from build123d import *

# Parameters (mm, degrees)
F1_DEPTH = 1.2
F2_DEPTH = 4
F3_DEPTH = 3.5
F4_W     = 1.7
F4_H     = 3.5
F5_DEPTH = 0.2


# Not quite as in the source:
# - a feature names something its author has since deleted; it is built from what else it names


with BuildPart() as f1:
    # F0 (on Top) → F1 (new body)
    with BuildSketch(Plane.XY):
        with BuildLine():
            ThreePointArc((-10.7121426428, 2.5), (-10.5820537772, 3.0033544341), (-10.4283268073, 3.5))
            Line((-10.4283268073, 3.5), (-14.25, 3.5))
            Line((-14.25, 3.5), (-14.25, 2.5))
            Line((-14.25, 2.5), (-10.7121426428, 2.5))
        make_face()
        with BuildLine():
            ThreePointArc((-10.4283268073, -3.5), (-10.5820537772, -3.0033544341), (-10.7121426428, -2.5))
            Line((-10.7121426428, -2.5), (-14.25, -2.5))
            Line((-14.25, -2.5), (-14.25, -3.5))
            Line((-14.25, -3.5), (-10.4283268073, -3.5))
        make_face()
        with BuildLine():
            Line((-9.3722996111, -2.5), (-10.7121426428, -2.5))
            ThreePointArc((-10.7121426428, -2.5), (-10.5820537772, -3.0033544341), (-10.4283268073, -3.5))
            Line((-10.4283268073, -3.5), (-9.0465463023, -3.5))
            ThreePointArc((-9.0465463023, -3.5), (-9.2229860238, -3.004418214), (-9.3722996111, -2.5))
        make_face()
        with BuildLine():
            Line((-9.0465463023, 3.5), (-10.4283268073, 3.5))
            ThreePointArc((-10.4283268073, 3.5), (-10.5820537772, 3.0033544341), (-10.7121426428, 2.5))
            Line((-10.7121426428, 2.5), (-9.3722996111, 2.5))
            ThreePointArc((-9.3722996111, 2.5), (-9.2229860238, 3.004418214), (-9.0465463023, 3.5))
        make_face()
        with BuildLine():
            Line((-9.3722996111, 2.5), (-10.7121426428, 2.5))
            ThreePointArc((-10.7121426428, 2.5), (-11, 0), (-10.7121426428, -2.5))
            Line((-10.7121426428, -2.5), (-9.3722996111, -2.5))
            ThreePointArc((-9.3722996111, -2.5), (-9.7, 0), (-9.3722996111, 2.5))
        make_face()
        with BuildLine():
            ThreePointArc((9.0465463023, 3.5), (7.606386924, 6.0193752136), (5.4854352608, 8))
            Line((5.4854352608, 8), (5, 8))
            Line((5, 8), (3.5, 6.4))
            Line((3.5, 6.4), (-3.5, 6.4))
            Line((-3.5, 6.4), (-5, 8))
            Line((-5, 8), (-5.4854352608, 8))
            ThreePointArc((-5.4854352608, 8), (-7.606386924, 6.0193752136), (-9.0465463023, 3.5))
            Line((-9.0465463023, 3.5), (9.0465463023, 3.5))
        make_face()
        with BuildLine():
            ThreePointArc((9.3722996111, 2.5), (9.2229860238, 3.004418214), (9.0465463023, 3.5))
            Line((9.0465463023, 3.5), (-9.0465463023, 3.5))
            ThreePointArc((-9.0465463023, 3.5), (-9.2229860238, 3.004418214), (-9.3722996111, 2.5))
            ThreePointArc((-9.3722996111, 2.5), (-9.7, 0), (-9.3722996111, -2.5))
            ThreePointArc((-9.3722996111, -2.5), (-9.2229860238, -3.004418214), (-9.0465463023, -3.5))
            Line((-9.0465463023, -3.5), (9.0465463023, -3.5))
            ThreePointArc((9.0465463023, -3.5), (9.2229860238, -3.004418214), (9.3722996111, -2.5))
            ThreePointArc((9.3722996111, -2.5), (9.6177259845, -1.2606930182), (9.7, 0))
            ThreePointArc((9.7, 0), (9.6177259845, 1.2606930182), (9.3722996111, 2.5))
        make_face()
        with BuildLine():
            Line((-5.4854352608, 8), (-7.5498344353, 8))
            ThreePointArc((-7.5498344353, 8), (-9.2663946827, 5.9273880912), (-10.4283268073, 3.5))
            Line((-10.4283268073, 3.5), (-9.0465463023, 3.5))
            ThreePointArc((-9.0465463023, 3.5), (-7.606386924, 6.0193752136), (-5.4854352608, 8))
        make_face()
        with BuildLine():
            ThreePointArc((10.4283268073, 3.5), (9.2663946827, 5.9273880912), (7.5498344353, 8))
            Line((7.5498344353, 8), (5.4854352608, 8))
            ThreePointArc((5.4854352608, 8), (7.606386924, 6.0193752136), (9.0465463023, 3.5))
            Line((9.0465463023, 3.5), (10.4283268073, 3.5))
        make_face()
        with BuildLine():
            Line((14.25, 3.5), (10.4283268073, 3.5))
            ThreePointArc((10.4283268073, 3.5), (10.5820537772, 3.0033544341), (10.7121426428, 2.5))
            Line((10.7121426428, 2.5), (14.25, 2.5))
            Line((14.25, 2.5), (14.25, 3.5))
        make_face()
        with BuildLine():
            Line((14.25, -2.5), (10.7121426428, -2.5))
            ThreePointArc((10.7121426428, -2.5), (10.5820537772, -3.0033544341), (10.4283268073, -3.5))
            Line((10.4283268073, -3.5), (14.25, -3.5))
            Line((14.25, -3.5), (14.25, -2.5))
        make_face()
        with BuildLine():
            ThreePointArc((10.4283268073, -3.5), (10.5820537772, -3.0033544341), (10.7121426428, -2.5))
            Line((10.7121426428, -2.5), (9.3722996111, -2.5))
            ThreePointArc((9.3722996111, -2.5), (9.2229860238, -3.004418214), (9.0465463023, -3.5))
            Line((9.0465463023, -3.5), (10.4283268073, -3.5))
        make_face()
        with BuildLine():
            ThreePointArc((11, 0), (10.9277987049, 1.258258902), (10.7121426428, 2.5))
            Line((10.7121426428, 2.5), (9.3722996111, 2.5))
            ThreePointArc((9.3722996111, 2.5), (9.6177259845, 1.2606930182), (9.7, 0))
            ThreePointArc((9.7, 0), (9.6177259845, -1.2606930182), (9.3722996111, -2.5))
            Line((9.3722996111, -2.5), (10.7121426428, -2.5))
            ThreePointArc((10.7121426428, -2.5), (10.9277987049, -1.258258902), (11, 0))
        make_face()
        with BuildLine():
            ThreePointArc((10.7121426428, 2.5), (10.5820537772, 3.0033544341), (10.4283268073, 3.5))
            Line((10.4283268073, 3.5), (9.0465463023, 3.5))
            ThreePointArc((9.0465463023, 3.5), (9.2229860238, 3.004418214), (9.3722996111, 2.5))
            Line((9.3722996111, 2.5), (10.7121426428, 2.5))
        make_face()
        with BuildLine():
            ThreePointArc((7.5498344353, -8), (9.2663946827, -5.9273880912), (10.4283268073, -3.5))
            Line((10.4283268073, -3.5), (9.0465463023, -3.5))
            ThreePointArc((9.0465463023, -3.5), (7.606386924, -6.0193752136), (5.4854352608, -8))
            Line((5.4854352608, -8), (7.5498344353, -8))
        make_face()
        with BuildLine():
            Line((9.0465463023, -3.5), (-9.0465463023, -3.5))
            ThreePointArc((-9.0465463023, -3.5), (-7.606386924, -6.0193752136), (-5.4854352608, -8))
            Line((-5.4854352608, -8), (5.4854352608, -8))
            ThreePointArc((5.4854352608, -8), (7.606386924, -6.0193752136), (9.0465463023, -3.5))
        make_face()
        with BuildLine():
            Line((-9.0465463023, -3.5), (-10.4283268073, -3.5))
            ThreePointArc((-10.4283268073, -3.5), (-9.2663946827, -5.9273880912), (-7.5498344353, -8))
            Line((-7.5498344353, -8), (-5.4854352608, -8))
            ThreePointArc((-5.4854352608, -8), (-7.606386924, -6.0193752136), (-9.0465463023, -3.5))
        make_face()
        with BuildLine():
            ThreePointArc((-10.7121426428, -2.5), (-11, 0), (-10.7121426428, 2.5))
            Line((-10.7121426428, 2.5), (-14.25, 2.5))
            Line((-14.25, 2.5), (-14.25, -2.5))
            Line((-14.25, -2.5), (-10.7121426428, -2.5))
        make_face()
        with BuildLine():
            Line((14.25, 2.5), (10.7121426428, 2.5))
            ThreePointArc((10.7121426428, 2.5), (10.9277987049, 1.258258902), (11, 0))
            ThreePointArc((11, 0), (10.9277987049, -1.258258902), (10.7121426428, -2.5))
            Line((10.7121426428, -2.5), (14.25, -2.5))
            Line((14.25, -2.5), (14.25, 2.5))
        make_face()
    extrude(amount=-F1_DEPTH)

    # F0 (on Top) → F2 (join)
    with BuildSketch(Plane.XY):
        with BuildLine():
            Line((-5.4854352608, 8), (-7.5498344353, 8))
            ThreePointArc((-7.5498344353, 8), (-9.2663946827, 5.9273880912), (-10.4283268073, 3.5))
            Line((-10.4283268073, 3.5), (-9.0465463023, 3.5))
            ThreePointArc((-9.0465463023, 3.5), (-7.606386924, 6.0193752136), (-5.4854352608, 8))
        make_face()
        with BuildLine():
            Line((-9.0465463023, 3.5), (-10.4283268073, 3.5))
            ThreePointArc((-10.4283268073, 3.5), (-10.5820537772, 3.0033544341), (-10.7121426428, 2.5))
            Line((-10.7121426428, 2.5), (-9.3722996111, 2.5))
            ThreePointArc((-9.3722996111, 2.5), (-9.2229860238, 3.004418214), (-9.0465463023, 3.5))
        make_face()
        with BuildLine():
            Line((-9.3722996111, -2.5), (-10.7121426428, -2.5))
            ThreePointArc((-10.7121426428, -2.5), (-10.5820537772, -3.0033544341), (-10.4283268073, -3.5))
            Line((-10.4283268073, -3.5), (-9.0465463023, -3.5))
            ThreePointArc((-9.0465463023, -3.5), (-9.2229860238, -3.004418214), (-9.3722996111, -2.5))
        make_face()
        with BuildLine():
            Line((-9.0465463023, -3.5), (-10.4283268073, -3.5))
            ThreePointArc((-10.4283268073, -3.5), (-9.2663946827, -5.9273880912), (-7.5498344353, -8))
            Line((-7.5498344353, -8), (-5.4854352608, -8))
            ThreePointArc((-5.4854352608, -8), (-7.606386924, -6.0193752136), (-9.0465463023, -3.5))
        make_face()
        with BuildLine():
            ThreePointArc((7.5498344353, -8), (9.2663946827, -5.9273880912), (10.4283268073, -3.5))
            Line((10.4283268073, -3.5), (9.0465463023, -3.5))
            ThreePointArc((9.0465463023, -3.5), (7.606386924, -6.0193752136), (5.4854352608, -8))
            Line((5.4854352608, -8), (7.5498344353, -8))
        make_face()
        with BuildLine():
            ThreePointArc((10.4283268073, -3.5), (10.5820537772, -3.0033544341), (10.7121426428, -2.5))
            Line((10.7121426428, -2.5), (9.3722996111, -2.5))
            ThreePointArc((9.3722996111, -2.5), (9.2229860238, -3.004418214), (9.0465463023, -3.5))
            Line((9.0465463023, -3.5), (10.4283268073, -3.5))
        make_face()
        with BuildLine():
            ThreePointArc((10.4283268073, 3.5), (9.2663946827, 5.9273880912), (7.5498344353, 8))
            Line((7.5498344353, 8), (5.4854352608, 8))
            ThreePointArc((5.4854352608, 8), (7.606386924, 6.0193752136), (9.0465463023, 3.5))
            Line((9.0465463023, 3.5), (10.4283268073, 3.5))
        make_face()
        with BuildLine():
            ThreePointArc((10.7121426428, 2.5), (10.5820537772, 3.0033544341), (10.4283268073, 3.5))
            Line((10.4283268073, 3.5), (9.0465463023, 3.5))
            ThreePointArc((9.0465463023, 3.5), (9.2229860238, 3.004418214), (9.3722996111, 2.5))
            Line((9.3722996111, 2.5), (10.7121426428, 2.5))
        make_face()
    extrude(amount=F2_DEPTH)

    # F0 (on Top) → F3 (join)
    with BuildSketch(Plane.XY):
        with BuildLine():
            ThreePointArc((-10.7121426428, 2.5), (-10.5820537772, 3.0033544341), (-10.4283268073, 3.5))
            Line((-10.4283268073, 3.5), (-14.25, 3.5))
            Line((-14.25, 3.5), (-14.25, 2.5))
            Line((-14.25, 2.5), (-10.7121426428, 2.5))
        make_face()
        with BuildLine():
            ThreePointArc((-10.4283268073, -3.5), (-10.5820537772, -3.0033544341), (-10.7121426428, -2.5))
            Line((-10.7121426428, -2.5), (-14.25, -2.5))
            Line((-14.25, -2.5), (-14.25, -3.5))
            Line((-14.25, -3.5), (-10.4283268073, -3.5))
        make_face()
        with BuildLine():
            Line((14.25, -2.5), (10.7121426428, -2.5))
            ThreePointArc((10.7121426428, -2.5), (10.5820537772, -3.0033544341), (10.4283268073, -3.5))
            Line((10.4283268073, -3.5), (14.25, -3.5))
            Line((14.25, -3.5), (14.25, -2.5))
        make_face()
        with BuildLine():
            Line((14.25, 3.5), (10.4283268073, 3.5))
            ThreePointArc((10.4283268073, 3.5), (10.5820537772, 3.0033544341), (10.7121426428, 2.5))
            Line((10.7121426428, 2.5), (14.25, 2.5))
            Line((14.25, 2.5), (14.25, 3.5))
        make_face()
    extrude(amount=F3_DEPTH)

    # F4 (on face) → F5 (join)
    with BuildSketch(Plane(origin=(0, 0, -1.2), x_dir=(1, 0, 0), z_dir=(0, 0, -1))):
        with Locations((-15.1, 0)):
            Rectangle(F4_W, F4_H)
        with Locations((15.1, 0)):
            Rectangle(F4_W, F4_H)
    extrude(amount=-F5_DEPTH)


solid = f1.part
Geometry: final body of the model. Coordinates: model frame, mm. A direction names the side the tool comes from. Give positions to 0.01 mm unless a question says otherwise; leave off trailing zeros. Order: outer loops, then holes, each group sorted by start corner. A loop starts at its lowest first (then second) coordinate and runs counter-clockwise, first axis right, second up. Notation, with made-up numbers: (25, 80) -> (66, 80) arc R20 ccw to (66, 98) -> close; hole circle Ø3 at (29, 51.5). An arc over 180 degrees is marked (long way). Put each result on its own line as item: value.
Q1. Reachability of faces 1 (the face through (12, -2.5, 2)), 2 (the face through (-12, -3.5, 1)), 3 (the face through (-7.95, 5.56, 1.97)), 4 (the face through (12, -3.5, 1)) from +Z, -Z, +X, -X, +Y, -Y: full face, straight path, thin tool, end or side. Return the list, or none.
Here are the results:
face 1: +Z, +X, -X
face 2: +Z, -Z, -X, -Y
face 3: +Z
face 4: +Z, -Z, +X, -Y
Q2. Section D-D, the plane y = -0.5. Return loops of the section in (x, z), then the cut area to 3 significant figures.
Here are the results:
outline: (-15.95, -1.2) -> (15.95, -1.2) -> (15.95, -1) -> (14.25, -1) -> (14.25, 0) -> (-14.25, 0) -> (-14.25, -1) -> (-15.95, -1) -> close
area: 34.9 mm^2
Q3. Draft query along X for faces 5 (the face through (0, 6.4, -1)), 6 (the face through (15, 0, -1)). Return one class per face: released by +X, released by -X, zero draft, split by the parting line, or undercut.
Here are the results:
face 5: undercut
face 6: zero draft
Q4. Material intervals for L1, parallel to Z at x = -4, y = -5.5; L2, parallel to Y at x = -12, z = -0.85; L3, parallel to X at y = 4.75, z = 2, sorted ascending.
Here are the results:
L1: z = -1.2 to 0
L2: y = -3.5 to 3.5
L3: x = -9.92 to -8.46, 8.46 to 9.92
Q5. Section C-C, the plane x = -8. Return loops of the section in (y, z).
Here are the results:
outline: (-7.55, -1.2) -> (7.55, -1.2) -> (7.55, 4) -> (5.49, 4) -> (5.49, 0) -> (-5.49, 0) -> (-5.49, 4) -> (-7.55, 4) -> close
Q6. Section B-B, the plane y = 7.25. Return loops of the section in (x, z), then the cut area to 3 significant figures.
Here are the results:
outline: (-8.27, -1.2) -> (-4.3, -1.2) -> (-4.3, 0) -> (-6.44, 0) -> (-6.44, 4) -> (-8.27, 4) -> close; (4.3, -1.2) -> (8.27, -1.2) -> (8.27, 4) -> (6.44, 4) -> (6.44, 0) -> (4.3, 0) -> close
area: 24.2 mm^2
Q7. Pin query (flat end, axial travel): pin 1 (3 mm diameter, centred on x = 12.5, z = 2, fed in from +Y); pin 2 (1.1 mm diameter, centred on x = 12.5, y = 3, fed in from +Z); pin 3 (3 mm diameter, centred on x = -2.5, z = 0.5, fed in from +Y); pin 4 (5 mm diameter, centred on x = 7, y = -6, fed in from +Z). Return the tip coordinate at first contact, or that it passes through.
Here are the results:
pin 1: stops at y = 3.5
pin 2: stops at z = 3.5
pin 3: stops at y = 6.84
pin 4: stops at z = 4
Q8. Section A-A, the plane z = 1.05. Return loops of the section in (x, y), then the cut area to 3 significant figures.
Here are the results:
outline: (-14.25, -3.5) -> (-10.43, -3.5) arc R11 ccw to (-7.55, -8) -> (-5.49, -8) arc R9.7 cw to (-9.37, -2.5) -> (-14.25, -2.5) -> close; (-14.25, 2.5) -> (-9.37, 2.5) arc R9.7 cw to (-5.49, 8) -> (-7.55, 8) arc R11 ccw to (-10.43, 3.5) -> (-14.25, 3.5) -> close; (5.49, -8) -> (7.55, -8) arc R11 ccw to (10.43, -3.5) -> (14.25, -3.5) -> (14.25, -2.5) -> (9.37, -2.5) arc R9.7 cw to start; (5.49, 8) arc R9.7 cw to (9.37, 2.5) -> (14.25, 2.5) -> (14.25, 3.5) -> (10.43, 3.5) arc R11 ccw to (7.55, 8) -> close
area: 49.2 mm^2
